Source: CAD feature listing. Evaluate the final solid. Frame: model axes, mm. Face numbers are marked on the shaded views. A direction names the side the tool comes from. Give positions to 0.01 mm unless a question says otherwise; leave off trailing zeros. Write each loop counter-clockwise with the first axis right and the second up, starting at its lowest first coordinate (ties: lowest second). Pieces come first, ordered by that corner, then holes.
```python
from build123d import *

# Parameters (mm, degrees)
SKETCH_1_W              = 25
SKETCH_1_H              = 1
SKETCH_2_R              = 22.55
EXTRUDE_1_DEPTH         = 6
SKETCH_3_W              = 4
SKETCH_3_H              = 1.5
SKETCH_4_W              = 4
SKETCH_4_H              = 1.5
SKETCH_5_W              = 4
SKETCH_5_H              = 1.5
SKETCH_6_W              = 4
SKETCH_6_H              = 1.5
SKETCH_7_W              = 4
SKETCH_7_H              = 1.5
SKETCH_8_W              = 4
SKETCH_8_H              = 1.5
HOLE_WIZARD_M24_1_D     = 26.12
HOLE_WIZARD_M24_1_DEPTH = 8.5
SKETCH_17_R             = 22.55
CUT_EXTRUDE_1_DEPTH     = 2.5


with BuildPart() as part:
    # 草图1 → 旋转1 (revolve)
    with BuildSketch(Plane(origin=(0, 0, 0), x_dir=(1, 0, 0), z_dir=(0, 1, 0))):
        with Locations((12.5, 22.5)):
            Rectangle(SKETCH_1_W, SKETCH_1_H)
    revolve(axis=Axis((0, 0, -23), (0, 0, 1)))

    # 草图2 → 凸台-拉伸1 (add)
    with BuildSketch(Plane(origin=(0, 0, -23), x_dir=(-1, 0, 0), z_dir=(0, 0, -1))):
        Circle(SKETCH_2_R)
    extrude(amount=EXTRUDE_1_DEPTH)

    # 草图3 → 旋转2 (revolve)
    with BuildSketch(Plane.XZ.offset(14.722431864)):
        with Locations((10.5, -21.25)):
            Rectangle(SKETCH_3_W, SKETCH_3_H)
    revolve(axis=Axis((8.5, -14.722431864, -20.5), (0, 0, -1)))

    # 草图4 → 旋转3 (revolve)
    with BuildSketch(Plane.XZ.offset(14.722431864)):
        with Locations((-6.5, -21.25)):
            Rectangle(SKETCH_4_W, SKETCH_4_H)
    revolve(axis=Axis((-8.5, -14.722431864, -20.5), (0, 0, -1)))

    # 草图5 → 旋转4 (revolve)
    with BuildSketch(Plane.XZ):
        with Locations((-15, -21.25)):
            Rectangle(SKETCH_5_W, SKETCH_5_H)
    revolve(axis=Axis((-17, 0, -20.5), (0, 0, -1)))

    # 草图6 → 旋转5 (revolve)
    with BuildSketch(Plane.XZ.offset(-14.722431864)):
        with Locations((-6.5, -21.25)):
            Rectangle(SKETCH_6_W, SKETCH_6_H)
    revolve(axis=Axis((-8.5, 14.722431864, -20.5), (0, 0, -1)))

    # 草图7 → 旋转6 (revolve)
    with BuildSketch(Plane.XZ.offset(-14.722431864)):
        with Locations((10.5, -21.25)):
            Rectangle(SKETCH_7_W, SKETCH_7_H)
    revolve(axis=Axis((8.5, 14.722431864, -20.5), (0, 0, -1)))

    # 草图8 → 旋转7 (revolve)
    with BuildSketch(Plane.XZ):
        with Locations((19, -21.25)):
            Rectangle(SKETCH_8_W, SKETCH_8_H)
    revolve(axis=Axis((17, 0, -20.5), (0, 0, -1)))

    # 草图9 → 切除-旋转1 (revolve, cut)
    with BuildSketch(Plane.XZ.offset(14.722431864)):
        Polygon((11.58, -20.5), (8.5, -20.5), (8.5, -29), (10.75, -29), (10.75, -23), (10.2, -23), (10.2, -22), (11.58, -22), align=None)
    revolve(axis=Axis((8.5, -14.722431864, -20.5), (0, 0, -1)), mode=Mode.SUBTRACT)

    # 草图10 → 切除-旋转2 (revolve, cut)
    with BuildSketch(Plane.XZ.offset(14.722431864)):
        Polygon((-5.42, -20.5), (-8.5, -20.5), (-8.5, -29), (-6.25, -29), (-6.25, -23), (-6.8, -23), (-6.8, -22), (-5.42, -22), align=None)
    revolve(axis=Axis((-8.5, -14.722431864, -20.5), (0, 0, -1)), mode=Mode.SUBTRACT)

    # 草图11 → 切除-旋转3 (revolve, cut)
    with BuildSketch(Plane.XZ):
        Polygon((-13.92, -20.5), (-17, -20.5), (-17, -29), (-14.75, -29), (-14.75, -23), (-15.3, -23), (-15.3, -22), (-13.92, -22), align=None)
    revolve(axis=Axis((-17, 0, -20.5), (0, 0, -1)), mode=Mode.SUBTRACT)

    # 草图12 → 切除-旋转4 (revolve, cut)
    with BuildSketch(Plane.XZ.offset(-14.722431864)):
        Polygon((-5.42, -20.5), (-8.5, -20.5), (-8.5, -29), (-6.25, -29), (-6.25, -23), (-6.8, -23), (-6.8, -22), (-5.42, -22), align=None)
    revolve(axis=Axis((-8.5, 14.722431864, -20.5), (0, 0, -1)), mode=Mode.SUBTRACT)

    # 草图13 → 切除-旋转5 (revolve, cut)
    with BuildSketch(Plane.XZ.offset(-14.722431864)):
        Polygon((11.58, -20.5), (8.5, -20.5), (8.5, -29), (10.75, -29), (10.75, -23), (10.2, -23), (10.2, -22), (11.58, -22), align=None)
    revolve(axis=Axis((8.5, 14.722431864, -20.5), (0, 0, -1)), mode=Mode.SUBTRACT)

    # 草图14 → 切除-旋转6 (revolve, cut)
    with BuildSketch(Plane.XZ):
        Polygon((20.08, -20.5), (17, -20.5), (17, -29), (19.25, -29), (19.25, -23), (18.7, -23), (18.7, -22), (20.08, -22), align=None)
    revolve(axis=Axis((17, 0, -20.5), (0, 0, -1)), mode=Mode.SUBTRACT)

    # M24 间隙孔1
    with Locations(Plane(origin=(0, 0, -29), x_dir=(-1, 0, 0), z_dir=(0, 0, -1))):
        with Locations((0, 0)):
            Hole(HOLE_WIZARD_M24_1_D / 2, depth=HOLE_WIZARD_M24_1_DEPTH)

    # 草图17 → 切除-拉伸1 (cut)
    with BuildSketch(Plane(origin=(0, 0, -29), x_dir=(-1, 0, 0), z_dir=(0, 0, -1))):
        Circle(SKETCH_17_R)
    extrude(amount=-CUT_EXTRUDE_1_DEPTH, mode=Mode.SUBTRACT)


solid = part.part
```
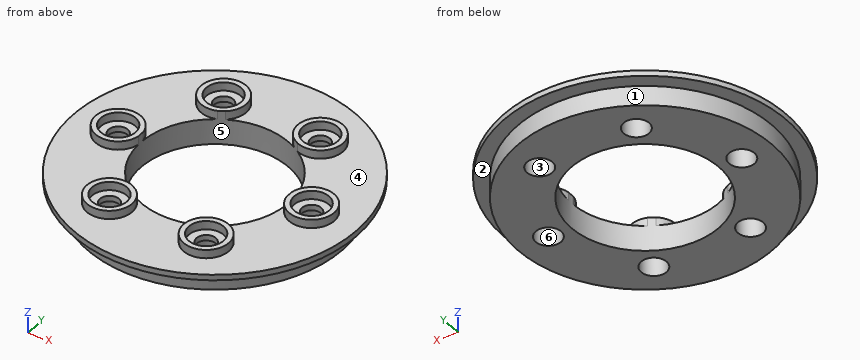
1. Pin query (flat end, axial travel): P1, Ø2, axis at x = 8, y = 15.5, coming from the -Z side; P2, Ø4.5, axis at x = 17, y = 0, coming from the +Z side; P3, Ø1.3, axis at x = -16.5, y = -0.5, coming from the -Z side; P4, Ø2, axis at y = -15.5, z = -23, coming from the -X side. Return the tip coordinate at first contact, or that it passes through.
2. Line query: probe 1 along X at (y, z) = (1, -21); probe 2 along Y at (x, z) = (17, -21.3); probe 3 along Y at (x, z) = (8.5, -21.5). Output: solid intervals per line, ascending.
3. Access query for the marked faces 4, 5 and 6. Directions: +Z, -Z, +X, -X, +Y, -Y. A direction counts if a zero-diameter tool reaches every point of the face in a straight line with its end or side. Return the directions, or none.
4. Section query D-D (z = -24.05). Return loops of the section in (x, y).
5. Section query C-C (y = -5). Return loops of the section in (x, z), plus the area to 3 significant figures.
6. Section query B-B (z = -21.4). Give the number of separate pieces and of enclosed holes in the cut face, plus the area to 3 significant figures.
7. Pull-direction query (Y, two-part tool) for the marked faces 1, 2 and 3; classes: pulls with the +Y half, pulls with the -Y half, needs draft (parallel to the pull), parting line crosses it, or undercut.
8. Section query A-A (x = 0). Return loops of the section in (y, z).
The answers:
1. P1: stops at z = -23
1. P2: stops at z = -22
1. P3: passes through
1. P4: stops at x = -20.37
2. probe 1: x = -20.87 to -19.91, -14.09 to -13.13, 13.13 to 14.09, 19.91 to 20.87
2. probe 2: y = -4 to -3.08, 3.08 to 4
2. probe 3: y = -18.72 to -17.8, -11.64 to -10.72, 10.72 to 11.64, 17.8 to 18.72
3. face 4: +Z
3. face 5: +Z, -Z
3. face 6: -Z
4. outline: circle Ø45.1 at (0, 0); hole circle Ø4.5 at (-17, 0); hole circle Ø26.12 at (0, 0); hole circle Ø4.5 at (-8.5, -14.72); hole circle Ø4.5 at (-8.5, 14.72); hole circle Ø4.5 at (8.5, -14.72); hole circle Ø4.5 at (8.5, 14.72); hole circle Ø4.5 at (17, 0)
5. outline: (-24.49, -23) - (-21.99, -23) - (-21.99, -26.5) - (-12.06, -26.5) - (-12.06, -22) - (-24.49, -22) - close; (12.06, -26.5) - (21.99, -26.5) - (21.99, -23) - (24.49, -23) - (24.49, -22) - (12.06, -22) - close
5. area: 94.3 mm2
6. separate pieces: 6
6. enclosed holes: 6
6. area: 122 mm2
7. face 1: parting line crosses it
7. face 2: needs draft
7. face 3: undercut
8. outline: (-25, -23) - (-22.55, -23) - (-22.55, -26.5) - (-13.06, -26.5) - (-13.06, -22) - (-25, -22) - close; (13.06, -26.5) - (22.55, -26.5) - (22.55, -23) - (25, -23) - (25, -22) - (13.06, -22) - close
